Check sheet for the modelled part. Datum: model origin and axes. Units: mm. Face numbers are marked on the shaded views. Round coordinates to 2 decimals unless told otherwise and drop trailing zeros. Return JSON: item names as keys, results as strings.
from build123d import *

# Parameters (mm, degrees)
SKETCH1_W          = 110.9726
SKETCH1_H          = 61.4426
EXTRUDE1_DEPTH     = 126.238
EXTRUDE1_DRAFT     = -0.3
CUT_EXTRUDE1_DEPTH = 3.175
CUT_EXTRUDE2_DEPTH = 12.7
SKETCH10_R         = 8.994906853
CUT_EXTRUDE3_DEPTH = 12.7
FILLET1_R          = 2.54
FILLET2_R          = 1.27
SKETCH2_R          = 2.0701
EXTRUDE2_DEPTH     = 1.016


with BuildPart() as part:
    # Sketch1 → Extrude1 (with draft: the straight prism first)
    with BuildSketch(Plane(origin=(0, 0, 0), x_dir=(1, 0, 0), z_dir=(0, 1, 0))):
        Rectangle(SKETCH1_W, SKETCH1_H)
    extrude(amount=-EXTRUDE1_DEPTH)
    # Extrude1: the draft: its side faces are tilted about the plane it starts from
    extrude1_sides = [part.faces().sort_by_distance(p)[0] for p in [
        (-55.4863, -63.119, 0),
        (0, -63.119, 30.7213),
        (55.4863, -63.119, 0),
        (0, -63.119, -30.7213),
    ]]
    draft(extrude1_sides, Plane(origin=(0, 0, 0), x_dir=(1, 0, 0), z_dir=(0, 1, 0)), EXTRUDE1_DRAFT)

    # Sketch9 → Cut-Extrude1 (cut)
    with BuildSketch(Plane(origin=(0, 0, 0), x_dir=(1, 0, 0), z_dir=(0, 1, 0))):
        with BuildLine():
            Line((-25.255419616, -1.4097), (-47.617180384, -1.4097))
            ThreePointArc((-47.617180384, -1.4097), (-48.960767849, -0.853167849), (-49.5173, 0.490419616))
            Line((-49.5173, 0.490419616), (-49.5173, 22.852180384))
            ThreePointArc((-49.5173, 22.852180384), (-48.960767849, 24.195767849), (-47.617180384, 24.7523))
            Line((-47.617180384, 24.7523), (-25.255419616, 24.7523))
            ThreePointArc((-25.255419616, 24.7523), (-23.911832151, 24.195767849), (-23.3553, 22.852180384))
            Line((-23.3553, 22.852180384), (-23.3553, 0.490419616))
            ThreePointArc((-23.3553, 0.490419616), (-23.911832151, -0.853167849), (-25.255419616, -1.4097))
        make_face()
    extrude(amount=-CUT_EXTRUDE1_DEPTH, mode=Mode.SUBTRACT)

    # Sketch9_3 → Cut-Extrude2 (cut)
    with BuildSketch(Plane(origin=(0, 0, 0), x_dir=(1, 0, 0), z_dir=(0, 1, 0))):
        with BuildLine():
            Line((-27.249309248, 6.419011382), (-23.3553, 6.419011382))
            Line((-23.3553, 6.419011382), (-23.3553, 22.852180384))
            ThreePointArc((-23.3553, 22.852180384), (-23.911832151, 24.195767849), (-25.255419616, 24.7523))
            Line((-25.255419616, 24.7523), (-43.215910219, 24.7523))
            Line((-43.215910219, 24.7523), (-43.215910219, 19.79682891))
            ThreePointArc((-43.215910219, 19.79682891), (-31.950614927, 21.255973402), (-25.853893147, 11.6713))
            ThreePointArc((-25.853893147, 11.6713), (-26.208694985, 8.954053148), (-27.249309248, 6.419011382))
        make_face()
        with BuildLine():
            Line((-47.617180384, -1.4097), (-31.184011382, -1.4097))
            Line((-31.184011382, -1.4097), (-31.184011382, 2.484309248))
            ThreePointArc((-31.184011382, 2.484309248), (-44.547832783, 4.874950192), (-44.56182891, 18.450910219))
            Line((-44.56182891, 18.450910219), (-49.5173, 18.450910219))
            Line((-49.5173, 18.450910219), (-49.5173, 0.490419616))
            ThreePointArc((-49.5173, 0.490419616), (-48.960767849, -0.853167849), (-47.617180384, -1.4097))
        make_face()
    extrude(amount=-CUT_EXTRUDE2_DEPTH, mode=Mode.SUBTRACT)

    # Sketch10 → Cut-Extrude3 (cut)
    with BuildSketch(Plane(origin=(0, -3.175, 0), x_dir=(1, 0, 0), z_dir=(0, 1, 0))):
        with Locations(Location((-36.4363, 11.6713, 0), (0, 0, 270))):
            Circle(SKETCH10_R)
        with BuildLine():
            Line((-35.6743, 18.737414212), (-35.6743, 17.975414212))
            ThreePointArc((-35.6743, 17.975414212), (-31.684395119, 15.883413484), (-30.0863, 11.6713))
            ThreePointArc((-30.0863, 11.6713), (-30.152493141, 10.756821264), (-30.349692554, 9.861407793))
            Line((-30.349692554, 9.861407793), (-29.622896406, 9.596875629))
            Line((-29.622896406, 9.596875629), (-29.883515756, 8.880829852))
            Line((-29.883515756, 8.880829852), (-30.610311903, 9.145362016))
            ThreePointArc((-30.610311903, 9.145362016), (-35.061908451, 5.471820355), (-40.648930859, 6.919853773))
            Line((-40.648930859, 6.919853773), (-41.195835744, 6.372948889))
            Line((-41.195835744, 6.372948889), (-41.734651111, 6.911764256))
            Line((-41.734651111, 6.911764256), (-41.187746227, 7.458669141))
            ThreePointArc((-41.187746227, 7.458669141), (-42.068818791, 8.739196306), (-42.612402774, 10.195408906))
            Line((-42.612402774, 10.195408906), (-43.374092784, 10.061102407))
            Line((-43.374092784, 10.061102407), (-43.506412695, 10.811525914))
            Line((-43.506412695, 10.811525914), (-42.744722686, 10.945832414))
            ThreePointArc((-42.744722686, 10.945832414), (-41.421425305, 15.604622476), (-37.1983, 17.975414212))
            Line((-37.1983, 17.975414212), (-37.1983, 18.737414212))
            Line((-37.1983, 18.737414212), (-35.6743, 18.737414212))
        make_face(mode=Mode.SUBTRACT)
    extrude(amount=-CUT_EXTRUDE3_DEPTH, mode=Mode.SUBTRACT)

    # Fillet1
    fillet1_edges = [part.edges().sort_by_distance(p)[0] for p in [
        (54.825313337, -126.238, 0),
        (0, -126.238, -30.060313337),
        (-54.825313337, -126.238, 0),
        (0, -126.238, 30.060313337),
        (-55.155806669, -63.119, -30.390806669),
        (55.155806669, -63.119, -30.390806669),
        (55.155806669, -63.119, 30.390806669),
        (-55.155806669, -63.119, 30.390806669),
    ]]
    fillet(fillet1_edges, radius=FILLET1_R)

    # Fillet2
    fillet2_edges = [part.edges().sort_by_distance(p)[0] for p in [
        (0, 0, 30.7213),
        (55.4863, 0, 0),
        (0, 0, -30.7213),
        (-55.4863, 0, 0),
        (54.742365646, 0, 29.977365646),
        (54.742365646, 0, -29.977365646),
        (-54.742365646, 0, 29.977365646),
        (-54.742365646, 0, -29.977365646),
        (-36.4363, 0, 1.4097),
        (-48.960767849, 0, 0.853167849),
        (-49.5173, 0, -11.6713),
        (-23.911832151, 0, -24.195767849),
        (-36.4363, 0, -24.7523),
        (-48.960767849, 0, -24.195767849),
        (-23.911832151, 0, 0.853167849),
        (-23.3553, 0, -11.6713),
    ]]
    fillet(fillet2_edges, radius=FILLET2_R)

    # Sketch2 → Extrude2 (cut)
    with BuildSketch(Plane(origin=(0, 0, 0), x_dir=(1, 0, 0), z_dir=(0, 1, 0))):
        with Locations(Location((-44.3103, -13.7287, 0), (0, 0, 270))):
            Circle(SKETCH2_R)
        with Locations(Location((-28.5623, -13.7287, 0), (0, 0, 270))):
            Circle(SKETCH2_R)
        with Locations(Location((-41.7703, -24.2443, 0), (0, 0, 270))):
            Circle(SKETCH2_R)
        with Locations(Location((-15.1003, 23.1013, 0), (0, 0, 270))):
            Circle(SKETCH2_R)
        with Locations(Location((-15.1003, 17.3863, 0), (0, 0, 270))):
            Circle(SKETCH2_R)
        with Locations(Location((-15.1003, 11.6713, 0), (0, 0, 270))):
            Circle(SKETCH2_R)
        with Locations(Location((-15.1003, 0.2413, 0), (0, 0, 90))):
            Circle(SKETCH2_R)
        with Locations(Location((-15.1003, 5.9563, 0), (0, 0, 90))):
            Circle(SKETCH2_R)
    extrude(amount=-EXTRUDE2_DEPTH, mode=Mode.SUBTRACT)


solid = part.part
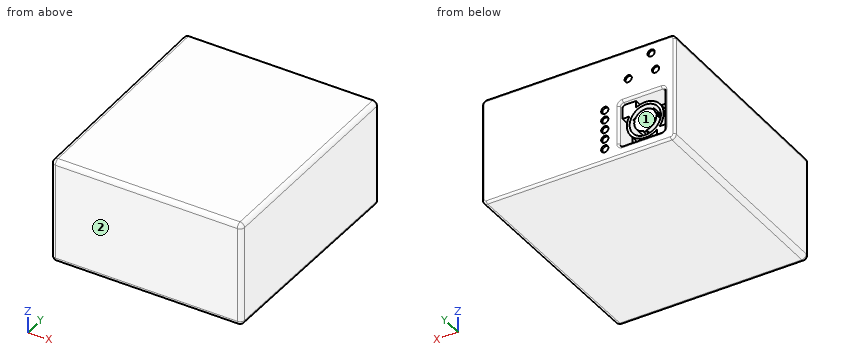
Q1. Material ranges on line 1 (X direction, y = -12.5, z = 22); line 2 (X direction, y = -57.5, z = -1); line 3 (Z direction, x = 11.5, y = -7.5), recorded low to high.
Results list:
{"line 1": "-55.42 to 55.42", "line 2": "-55.19 to 55.19", "line 3": "-30.68 to 30.68"}
Q2. Draft check along X on the marked faces 1 and 2. Enter one of: released by +X, released by -X, zero draft, split by the parting line, or undercut.
Results list:
{"face 1": "undercut", "face 2": "zero draft"}
Q3. Go/stop test with flat-tipped pins: pin 1 (1.5 mm diameter, centred on y = -10, z = -23, fed in from +X); pin 2 (8 mm diameter, centred on y = -56.5, z = -21, fed in from -X); pin 3 (0.6 mm diameter, centred on y = -7, z = -18, fed in from -X). Record where each tip stops, or that it passes through.
Results list:
{"pin 1": "x = 55.44", "pin 2": "x = -55.21", "pin 3": "x = -55.45"}
